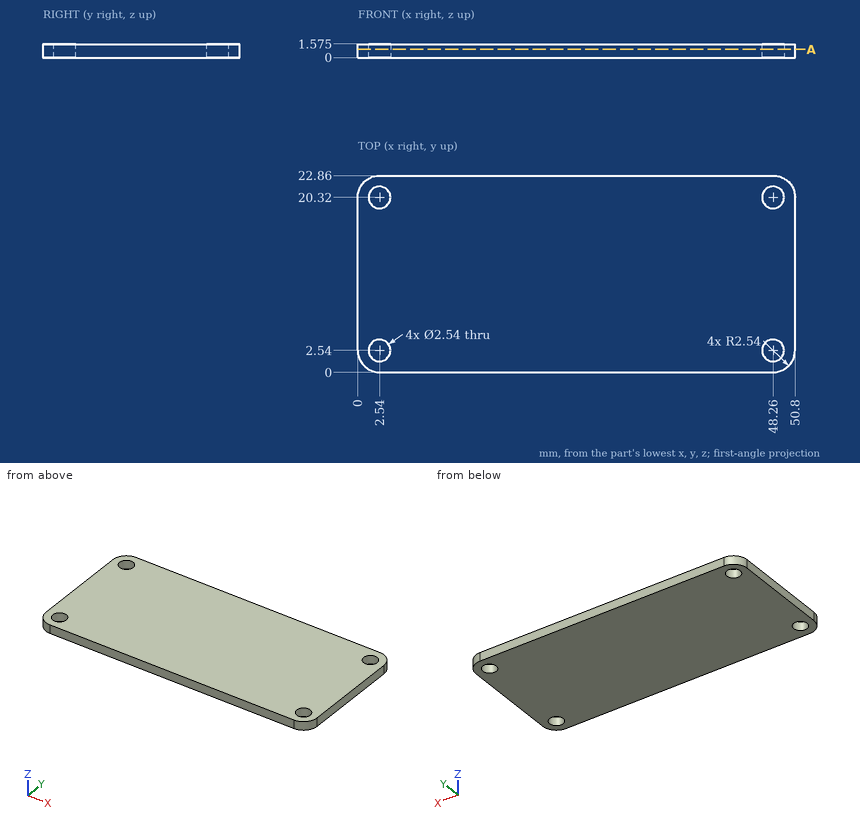
Part print with two shaded views. Sizes in mm from the minimum x, y, z corner. Round coordinates to 2 decimals unless told otherwise and drop trailing zeros. Write each loop counter-clockwise with the first axis right and the second up, starting at its lowest first coordinate (ties: lowest second). Pieces come first, ordered by that corner, then holes. Notation, with made-up numbers: M 77,31.25 L 131,31.25 A24 cw 131,62.25 Z; hole C 58,-37.75 d4. An arc over 180 degrees is marked long. Answer as CSV lines item,"result". Start each with the question number.
1) Band-saw the part on A-A (z = 0.95). List the corners of the cut face in (x, y).
2) Drill centre lines: L1, parallel to Y at x = 48.26, z = 0.45; L2, parallel to X at y = 2.5, z = 1. Where is each one in solid material? Low to high.
3) Drop flat-ended pins along their axis: pin 1 (3 mm diameter, centred on x = 41.5, y = 10, fed in from -Z); pin 2 (2 mm diameter, centred on x = 48.26, y = 20.32, fed in from +Z). Give the stop position or say it passes through.
Worked out:
1,outline,"M 0,2.54 A2.54 ccw 2.54,0 L 48.26,0 A2.54 ccw 50.8,2.54 L 50.8,20.32 A2.54 ccw 48.26,22.86 L 2.54,22.86 A2.54 ccw 0,20.32 Z; hole C 2.54,2.54 d2.54; hole C 2.54,20.32 d2.54; hole C 48.26,2.54 d2.54; hole C 48.26,20.32 d2.54"
2,L1,"0 to 1.27, 3.81 to 19.05, 21.59 to 22.86"
2,L2,"0 to 1.27, 3.81 to 46.99, 49.53 to 50.8"
3,pin 1,"z = 0"
3,pin 2,"through"
